```python
from build123d import *

# Parameters (mm, degrees)
BOSS_EXTRUDE1_DEPTH = 2.5
BOSS_EXTRUDE2_DEPTH = 2.5
SKETCH3_R           = 1.25
BOSS_EXTRUDE3_DEPTH = 2.5
SKETCH4_R           = 1.25
BOSS_EXTRUDE4_DEPTH = 2.5


with BuildPart() as part:
    # Sketch1 → Boss-Extrude1 (new body)
    with BuildSketch(Plane(origin=(0, 0, 0), x_dir=(1, 0, 0), z_dir=(0, 1, 0))):
        with BuildLine():
            Line((4, 6.75), (4, 0))
            ThreePointArc((4, 0), (0, -4), (-4, 0))
            Line((-4, 0), (-4, 6.75))
            ThreePointArc((-4, 6.75), (0, 10.75), (4, 6.75))
        make_face()
    extrude(amount=BOSS_EXTRUDE1_DEPTH)

    # Sketch1<3> → Boss-Extrude2 (add)
    with BuildSketch(Plane(origin=(0, 0, 0), x_dir=(1, 0, 0), z_dir=(0, 1, 0))):
        with BuildLine():
            Line((4, 6.75), (4, 0))
            ThreePointArc((4, 0), (0, -4), (-4, 0))
            Line((-4, 0), (-4, 6.75))
            ThreePointArc((-4, 6.75), (0, 10.75), (4, 6.75))
        make_face()
    extrude(amount=BOSS_EXTRUDE2_DEPTH)

    # Sketch3 → Boss-Extrude3 (add)
    with BuildSketch(Plane(origin=(0, 2.5, 0), x_dir=(1, 0, 0), z_dir=(0, 1, 0))):
        Circle(SKETCH3_R)
    extrude(amount=BOSS_EXTRUDE3_DEPTH)

    # Sketch4 → Boss-Extrude4 (add)
    with BuildSketch(Plane.XZ):
        with Locations((0, -6.75)):
            Circle(SKETCH4_R)
    extrude(amount=BOSS_EXTRUDE4_DEPTH)


solid = part.part
```
Check sheet for the modelled part. Datum: model origin and axes. Units: mm. A direction names the side the tool comes from. Round coordinates to 2 decimals unless told otherwise and drop trailing zeros. Order: outer loops, then holes, each group sorted by start corner. A loop starts at its lowest first (then second) coordinate and runs counter-clockwise, first axis right, second up. Notation, with made-up numbers: M 50,65.25 L 70,65.25 A23 ccw 70,90.25 Z; hole C 22.5,88 d11. An arc over 180 degrees is marked long. Answer in a Markdown table with one row per item.
(1) Section check D-D on x = -0.75. Record the boundary of the cut face in (y, z).
Findings:
| item | result |
|---|---|
| outline | M -2.5,-7.75 L 0,-7.75 L 0,-10.68 L 2.5,-10.68 L 2.5,-1 L 5,-1 L 5,1 L 2.5,1 L 2.5,3.93 L 0,3.93 L 0,-5.75 L -2.5,-5.75 Z |
(2) Gauge pin test, flat end, axial feed: pin 1 (1 mm diameter, centred on x = 3, y = 1.5, fed in from +Z). Record the tip position at first contact, or that the pin passes through.
Findings:
| item | result |
|---|---|
| pin 1 | stops at z = 3.12 |
(3) Set-up check for faces 1 (the flat face through (-4, 1, -3)), 2 (the cylindrical face through (-0.27, 3.73, 1.22)), 3 (the cylindrical face through (0, -1, -8)): record each of +Z, -Z, +X, -X, +Y, -Y from which the full face is reachable in a straight line by a thin tool's end or side.
Findings:
| item | result |
|---|---|
| face 1 | +Z, -Z, -X, +Y, -Y |
| face 2 | +Y |
| face 3 | -Y |
(4) Section check C-C on z = 0.5. Record the boundary of the cut face in (x, y), plus the area to 3 significant figures.
Findings:
| item | result |
|---|---|
| outline | M -3.97,0 L 3.97,0 L 3.97,2.5 L 1.15,2.5 L 1.15,5 L -1.15,5 L -1.15,2.5 L -3.97,2.5 Z |
| area | 25.6 mm^2 |
(5) Material ranges on line 1 along Z through (x, y) = (0, -1); line 2 along Y through (x, z) = (1, -3.75); line 3 along X through (y, z) = (1.25, 0.25), recorded low to high. Write a range as from..to.
Findings:
| item | result |
|---|---|
| line 1 | z = -8..-5.5 |
| line 2 | y = 0..2.5 |
| line 3 | x = -3.99..3.99 |
(6) Section check A-A on x = 0.25. Record the boundary of the cut face in (y, z), plus the area to 3 significant figures.
Findings:
| item | result |
|---|---|
| outline | M -2.5,-7.97 L 0,-7.97 L 0,-10.74 L 2.5,-10.74 L 2.5,-1.22 L 5,-1.22 L 5,1.22 L 2.5,1.22 L 2.5,3.99 L 0,3.99 L 0,-5.53 L -2.5,-5.53 Z |
| area | 49.1 mm^2 |
(7) Section check B-B on y = -0.25. Record the boundary of the cut face in (x, z).
Findings:
| item | result |
|---|---|
| outline | C 0,-6.75 d2.5 |
